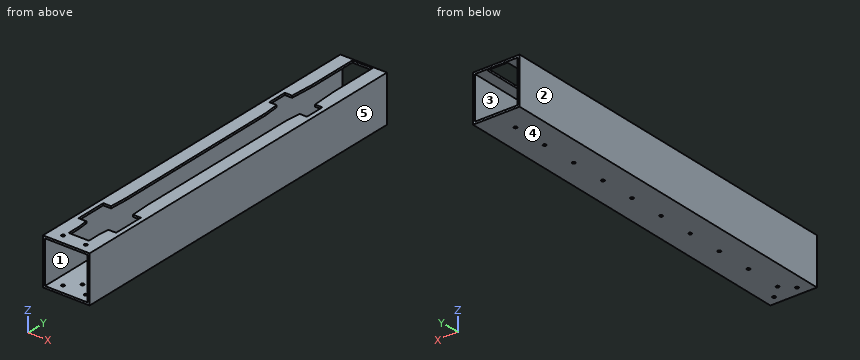
```python
from build123d import *

# Parameters (mm, degrees)
F0_W     = 76.2
F0_H     = 76.2
F0_W_2   = 69.596
F0_H_2   = 69.596
F1_DEPTH = 609.6
F3_DEPTH = 25.4
F5_D     = 5.08


with BuildPart() as f1:
    # F0 (on Front) → F1 (new body)
    with BuildSketch(Plane.XZ):
        with Locations((21.630452, 18.620882)):
            Rectangle(F0_W, F0_H)
        with Locations((21.630452, 18.620882)):
            Rectangle(F0_W_2, F0_H_2, mode=Mode.SUBTRACT)
    extrude(amount=F1_DEPTH)

    # F2 (on face) → F3 (cut)
    with BuildSketch(Plane.XY.offset(56.720882)):
        Polygon((38.140452, -2.54), (5.120452, -2.54), (5.120452, -83.82), (2.834452, -123.19), (-9.103548, -123.19), (-9.103548, -154.94), (2.834452, -154.94), (5.120452, -180.34), (5.120452, -467.36), (3.596452, -495.3), (-9.103548, -495.3), (-9.103548, -546.1), (3.596452, -546.1), (5.251717, -563.88), (5.251717, -584.2), (38.271717, -584.2), (38.271717, -563.88), (39.664452, -546.1), (52.364452, -546.1), (52.364452, -495.3), (39.664452, -495.3), (38.140452, -467.36), (38.140452, -180.34), (40.426452, -154.94), (52.364452, -154.94), (52.364452, -123.19), (40.426452, -123.19), (38.140452, -83.82), align=None)
    extrude(amount=-F3_DEPTH, mode=Mode.SUBTRACT)

    # F5 (through all)
    with Locations(Plane(origin=(0, 0, -19.479118), x_dir=(1, 0, 0), z_dir=(0, 0, -1))):
        with Locations((21.630452, 576.58), (21.630452, 516.89), (21.630452, 457.2), (21.630452, 397.51), (21.630452, 337.82), (21.630452, 278.13), (21.630452, 218.44), (21.630452, 158.75), (21.630452, 99.06), (21.630452, 39.37), (3.850452, 594.042182), (41.950452, 595.025122)):
            Hole(F5_D / 2)


solid = f1.part
```
Geometry check sheet. Reference: the model listing, model coordinates, mm. Face numbers are marked on the shaded views. A direction names the side the tool comes from. Coordinates: 2 decimals unless noted, no trailing zeros. Order: outer loops, then holes, each group sorted by start corner. A loop starts at its lowest first (then second) coordinate and runs counter-clockwise, first axis right, second up. Notation, with made-up numbers: M 5.25,89 L 59.25,89 A22 ccw 59.25,117 Z; hole C -10,20.25 d11. An arc over 180 degrees is marked long. One line per question, with ' | ' between items. Start each with the question number.
Item 1: Cross-section at C-C on y = -266. Enter the section's corners in (x, z), then the cut area to 3 significant figures.
Item 2: Set-up check for the marked faces 1 and 2: record each of +Z, -Z, +X, -X, +Y, -Y from which the full face is reachable in a straight line by a thin tool's end or side.
Item 3: Cross-section at D-D on y = -174. Enter the section's corners in (x, z).
Item 4: Material ranges on L1, parallel to X at y = -555.5, z = 37; L2, parallel to Z at x = 0.5, y = -116.5; L3, parallel to X at y = -39.37, z = -18.3, recorded low to high. Write a range as [from, to].
Item 5: Cross-section at A-A on z = -10.5. Enter the section's corners in (x, y), then the cut area to 3 significant figures.
Item 6: Gauge pin test, flat ends, axial feed: pin 1 (3 mm diameter, centred on x = 21.63, y = -397.51, fed in from -Z); pin 2 (2 mm diameter, centred on x = 22.5, y = -290.5, fed in from +Z). Record the tip position at first contact, or that the pin passes through.
Item 7: Cross-section at B-B on x = 33. Enter the section's corners in (y, z).
Item 8: Draft check along Z on the marked faces 3, 4 and 5. Enter one of: pulls with the +Z half, pulls with the -Z half, needs draft (parallel to the pull), parting line crosses it, or undercut.
Findings:
1) outline: M -16.47,-19.48 L 59.73,-19.48 L 59.73,56.72 L 38.14,56.72 L 38.14,53.42 L 56.43,53.42 L 56.43,-16.18 L -13.17,-16.18 L -13.17,53.42 L 5.12,53.42 L 5.12,56.72 L -16.47,56.72 Z | area: 854 mm²
2) face 1: +Y, -Y | face 2: +Z, -Z, -X, +Y, -Y
3) outline: M -16.47,-19.48 L 59.73,-19.48 L 59.73,56.72 L 38.71,56.72 L 38.71,53.42 L 56.43,53.42 L 56.43,-16.18 L -13.17,-16.18 L -13.17,53.42 L 4.55,53.42 L 4.55,56.72 L -16.47,56.72 Z
4) L1: x = [-16.47, -13.17], [56.43, 59.73] | L2: z = [-19.48, -16.18], [53.42, 56.72] | L3: x = [-16.47, 19.09], [24.17, 59.73]
5) outline: M -16.47,-609.6 L -13.17,-609.6 L -13.17,0 L -16.47,0 Z; M 56.43,-609.6 L 59.73,-609.6 L 59.73,0 L 56.43,0 Z | area: 4,030 mm²
6) pin 1: passes through | pin 2: stops at z = -16.18
7) outline: M -609.6,-19.48 L 0,-19.48 L 0,-16.18 L -609.6,-16.18 Z; M -609.6,53.42 L -584.2,53.42 L -584.2,56.72 L -609.6,56.72 Z; M -2.54,53.42 L 0,53.42 L 0,56.72 L -2.54,56.72 Z
8) face 3: undercut | face 4: pulls with the -Z half | face 5: needs draft
